Geometry check sheet. Reference: the model listing, model coordinates, mm. Give positions to 0.01 mm unless a question says otherwise; leave off trailing zeros. Order: outer loops, then holes, each group sorted by start corner. A loop starts at its lowest first (then second) coordinate and runs counter-clockwise, first axis right, second up.
from build123d import *

# Parameters (mm, degrees)
BASPROSKE_W           = 12
BASPROSKE_H           = 17.5
TOOTHCUT_DEPTH        = 28.504545079
TEETHCUTS_COUNT       = 12
TEETHCUTS_ANGLE       = 330
BORSKE_R              = 1.5
BORE_DEPTH            = 50.0000508
CROQUIS1_R            = 1.5875
CORTAR_EXTRUIR1_DEPTH = 27.88866135


with BuildPart() as part:
    # BasProSke → Base-Revolve (revolve)
    with BuildSketch(Plane(origin=(0, 0, 0), x_dir=(1, 0, 0), z_dir=(0, 1, 0)), mode=Mode.PRIVATE) as base_revolve_sk:
        with Locations((6, 8.75)):
            Rectangle(BASPROSKE_W, BASPROSKE_H)
    revolve(base_revolve_sk.sketch.rotate(Axis((-10, 0, 0), (1, 0, 0)), 180), axis=Axis((-10, 0, 0), (1, 0, 0)))

    # TooCutSke → ToothCut (cut, through all)
    with BuildSketch(Plane(origin=(0, 0, 0), x_dir=(0, 0, -1), z_dir=(1, 0, 0))):
        with BuildLine():
            ThreePointArc((1.394381134, 11.791843675), (0, 11.874), (-1.394381134, 11.791843675))
            ThreePointArc((-1.394381134, 11.791843675), (-2.068078374, 14.771857381), (-4.121860996, 17.033787221))
            ThreePointArc((-4.121860996, 17.033787221), (0, 17.5254), (4.121860996, 17.033787221))
            ThreePointArc((4.121860996, 17.033787221), (2.068078374, 14.771857381), (1.394381134, 11.791843675))
        make_face()
    toothcut = extrude(amount=TOOTHCUT_DEPTH, mode=Mode.SUBTRACT)

    # TeethCuts: ToothCut ×12 about axis
    teethcuts_axis = Axis((-10, 0, 0), (1, 0, 0))
    for i in range(1, TEETHCUTS_COUNT):
        add(toothcut.rotate(teethcuts_axis, i * TEETHCUTS_ANGLE / (TEETHCUTS_COUNT - 1)), mode=Mode.SUBTRACT)

    # BorSke → Bore (cut, symmetric)
    with BuildSketch(Plane(origin=(0, 0, 0), x_dir=(0, 0, -1), z_dir=(1, 0, 0))):
        with Locations(Location((0, 0, 0), (0, 0, 180))):
            Circle(BORSKE_R)
    extrude(amount=BORE_DEPTH, both=True, mode=Mode.SUBTRACT)

    # Croquis1 → Cortar-Extruir1 (cut, through all)
    with BuildSketch(Plane.ZY):
        Circle(CROQUIS1_R)
    extrude(amount=-CORTAR_EXTRUIR1_DEPTH, mode=Mode.SUBTRACT)


solid = part.part
Item 1: Scan lines: L1, parallel to Y at x = 11, z = 5; L2, parallel to Y at x = 8.5, z = 11; L3, parallel to Z at x = 3.25, y = 10. Record each from-to range of solid material in increasing order.
Reported:
L1: y = -16.71 to -11.47, -10.77 to 10.77, 11.47 to 16.71
L2: y = -12.53 to -8.22, -4.74 to 4.74, 8.22 to 12.53
L3: z = -12.2 to -7.39, -6.4 to 6.4, 7.39 to 12.2
Item 2: Sectioned sample at C-C (z = 3.5). Enter the section's corners in (x, y).
Reported:
outline: (0, -16.57) - (12, -16.57) - (12, 16.57) - (0, 16.57) - close
Item 3: Draft check along Z on faces 1 (the cylindrical face through (5.916, -10.273, 5.954)), 2 (the cylindrical face through (5.916, 10.293, 5.92)), 3 (the cylindrical face through (6.084, 4.523, -16.905)), 4 (the flat face through (12, -4, 0)). Enter one of: released by +Z, released by -Z, zero draft, split by the parting line, or undercut.
Reported:
face 1: undercut
face 2: undercut
face 3: released by -Z
face 4: zero draft
Item 4: Sectioned sample at D-D (y = -6.5). Enter the section's corners in (x, z), and give its area (3 significant figures).
Reported:
outline: (0, -9.94) - (12, -9.94) - (12, 9.94) - (0, 9.94) - close
area: 238 mm2
Item 5: Gauge pin test, flat ends, axial feed: pin 1 (1 mm diameter, centred on x = 7.5, z = 5, fed in from +Y); pin 2 (4 mm diameter, centred on x = 8, y = 13, fed in from +Z); pin 3 (2.5 mm diameter, centred on y = 0, z = 0, fed in from +X); pin 4 (1.5 mm diameter, centred on x = 9.5, z = -5.5, fed in from +Y). Record the tip position at first contact, or that the pin passes through.
Reported:
pin 1: stops at y = 16.91
pin 2: stops at z = 12.69
pin 3: passes through
pin 4: stops at y = 16.84
Item 6: Sectioned sample at A-A (y = 0). Enter the section's corners in (x, z).
Reported:
outline: (0, -11.87) - (12, -11.87) - (12, -1.59) - (0, -1.59) - close; (0, 1.59) - (12, 1.59) - (12, 11.87) - (0, 11.87) - close
